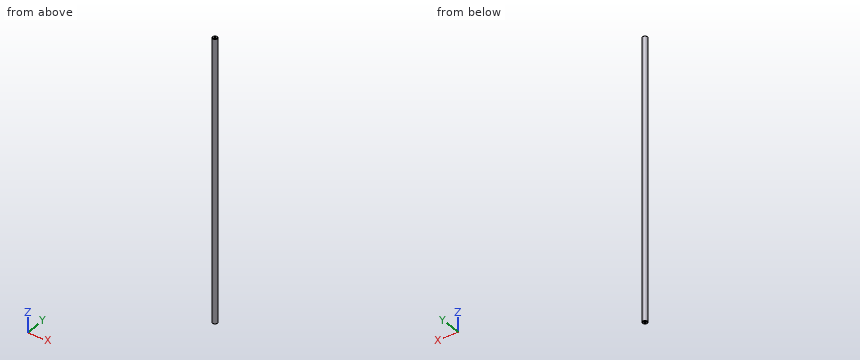
```python
from build123d import *

# Parameters (mm, degrees)
ESQUISSE1_R           = 4
BOSS_EXTRU_1_DEPTH    = 480
CHANFREIN1_SIZE       = 0.5
TROU_TARAUD_M41_D     = 3.3
TROU_TARAUD_M41_DEPTH = 11.5
TROU_TARAUD_M41_TIP   = 0.991420021
TROU_TARAUD_M42_D     = 3.3
TROU_TARAUD_M42_DEPTH = 11.5
TROU_TARAUD_M42_TIP   = 0.991420021


with BuildPart() as part:
    # Esquisse1 → Boss.-Extru.1 (new body)
    with BuildSketch(Plane.XY):
        Circle(ESQUISSE1_R)
    extrude(amount=BOSS_EXTRU_1_DEPTH)

    # Chanfrein1
    chanfrein1_edges = [part.edges().sort_by_distance(p)[0] for p in [
        (-4, 0, 0),
        (-4, 0, 480),
    ]]
    chamfer(chanfrein1_edges, length=CHANFREIN1_SIZE)

    # Trou taraudé M41
    with Locations(Plane.XY.offset(480)):
        with Locations((0, 0)):
            Hole(TROU_TARAUD_M41_D / 2, depth=TROU_TARAUD_M41_DEPTH)
            with Locations((0, 0, -(TROU_TARAUD_M41_DEPTH + TROU_TARAUD_M41_TIP / 2))):  # 118° drill point
                Cone(0, TROU_TARAUD_M41_D / 2, TROU_TARAUD_M41_TIP, mode=Mode.SUBTRACT)

    # Trou taraudé M42
    with Locations(Plane(origin=(0, 0, 0), x_dir=(-1, 0, 0), z_dir=(0, 0, -1))):
        with Locations((0, 0)):
            Hole(TROU_TARAUD_M42_D / 2, depth=TROU_TARAUD_M42_DEPTH)
            with Locations((0, 0, -(TROU_TARAUD_M42_DEPTH + TROU_TARAUD_M42_TIP / 2))):  # 118° drill point
                Cone(0, TROU_TARAUD_M42_D / 2, TROU_TARAUD_M42_TIP, mode=Mode.SUBTRACT)


solid = part.part
```
Work out the finished part from the listing and answer in its coordinate system (mm). Give positions to 0.01 mm unless a question says otherwise; leave off trailing zeros. Order: outer loops, then holes, each group sorted by start corner. A loop starts at its lowest first (then second) coordinate and runs counter-clockwise, first axis right, second up. Notation, with made-up numbers: (8.25, 87) - (61.25, 87) arc R17 cw to (61.25, 95) - close; hole circle Ø6 at (75, 44). An arc over 180 degrees is marked (long way). One line per item, written item: value. Start each with the question number.
1. Consider line 1 (Y direction, x = 0, z = 3.25); line 2 (Z direction, x = 0.5, y = -1.5); line 3 (X direction, y = 0.75, z = 458.5). Determine where each line is inside the solid, lowest interval first.
2. Section A-A, the plane z = 412 is taken. Write down the section's boundary in (x, y).
3. Each of these flat-tipped pins is pushed along its axis until it touches: pin 1 Ø1 at (x, z) = (3, 258.5) entering from +Y; pin 2 Ø4 at (y, z) = (-1, 189) entering from +X; pin 3 Ø1.5 at (y, z) = (1.5, 203) entering from -X; pin 4 Ø2.5 at (x, y) = (0, 0) entering from -Z. Where does it stop, or does it pass through?
Filled sheet:
1. line 1: -4 to -1.65, 1.65 to 4
1. line 2: 11.54 to 468.46
1. line 3: -3.93 to 3.93
2. outline: circle Ø8 at (0, 0)
3. pin 1: y = 3.12
3. pin 2: x = 4
3. pin 3: x = -3.93
3. pin 4: z = 11.74
